Read the model definition and answer for the solid it produces. Units are mm, in the model's axes. Give positions to 0.01 mm unless a question says otherwise; leave off trailing zeros. Order: outer loops, then holes, each group sorted by start corner. A loop starts at its lowest first (then second) coordinate and runs counter-clockwise, first axis right, second up. Notation, with made-up numbers: (38.25, 79.5) - (43.25, 79.5) arc R12 ccw to (43.25, 84.5) - close; hole circle Ø2 at (-18.75, 21.25). An arc over 180 degrees is marked (long way). Return JSON: item names as keys, results as strings.
```python
from build123d import *

# Parameters (mm, degrees)
F0_R     = 3.5
F0_W     = 5
F0_H     = 25
F1_DEPTH = 1


with BuildPart() as f1:
    # F0 (on Top) → F1 (new body)
    with BuildSketch(Plane.XY):
        with BuildLine():
            ThreePointArc((24.235588, 30.946928), (30.976758, 28.377192), (35.314001, 34.142193))
            ThreePointArc((35.314001, 34.142193), (31.334351, 39.791811), (24.674606, 37.946928))
            ThreePointArc((24.674606, 37.946928), (23.325767, 34.517756), (24.235588, 30.946928))
        make_face()
        with Locations((29.314001, 34.142193)):
            Circle(F0_R, mode=Mode.SUBTRACT)
        with BuildLine():
            ThreePointArc((24.235588, 30.946928), (23.325767, 34.517756), (24.674606, 37.946928))
            Line((24.674606, 37.946928), (0, 37.946928))
            Line((0, 37.946928), (-24.674606, 37.946928))
            ThreePointArc((-24.674606, 37.946928), (-23.664383, 36.162543), (-23.314001, 34.142193))
            ThreePointArc((-23.314001, 34.142193), (-23.549, 32.479436), (-24.235588, 30.946928))
            Line((-24.235588, 30.946928), (-4.218093, 30.946928))
            Line((-4.218093, 30.946928), (-4.218093, 20.946928))
            Line((-4.218093, 20.946928), (-14.650477, 20.946928))
            Line((-14.650477, 20.946928), (-14.650477, 0))
            Line((-14.650477, 0), (-14.650477, -20.946928))
            Line((-14.650477, -20.946928), (-4.218093, -20.946928))
            Line((-4.218093, -20.946928), (-4.218093, -30.946928))
            Line((-4.218093, -30.946928), (-24.235588, -30.946928))
            ThreePointArc((-24.235588, -30.946928), (-23.549, -32.479436), (-23.314001, -34.142193))
            ThreePointArc((-23.314001, -34.142193), (-23.664383, -36.162543), (-24.674606, -37.946928))
            Line((-24.674606, -37.946928), (0, -37.946928))
            Line((0, -37.946928), (24.674606, -37.946928))
            ThreePointArc((24.674606, -37.946928), (23.325767, -34.517756), (24.235588, -30.946928))
            Line((24.235588, -30.946928), (4.218093, -30.946928))
            Line((4.218093, -30.946928), (4.218093, -20.946928))
            Line((4.218093, -20.946928), (14.650477, -20.946928))
            Line((14.650477, -20.946928), (14.650477, 0))
            Line((14.650477, 0), (14.650477, 20.946928))
            Line((14.650477, 20.946928), (4.218093, 20.946928))
            Line((4.218093, 20.946928), (4.218093, 30.946928))
            Line((4.218093, 30.946928), (24.235588, 30.946928))
        make_face()
        with Locations((-4, 0)):
            Rectangle(F0_W, F0_H, mode=Mode.SUBTRACT)
        with Locations((4, 0)):
            Rectangle(F0_W, F0_H, mode=Mode.SUBTRACT)
        with BuildLine():
            ThreePointArc((-23.314001, 34.142193), (-23.664383, 36.162543), (-24.674606, 37.946928))
            ThreePointArc((-24.674606, 37.946928), (-35.302236, 33.76663), (-24.235588, 30.946928))
            ThreePointArc((-24.235588, 30.946928), (-23.549, 32.479436), (-23.314001, 34.142193))
        make_face()
        with Locations((-29.314001, 34.142193)):
            Circle(F0_R, mode=Mode.SUBTRACT)
        with BuildLine():
            ThreePointArc((35.314001, -34.142193), (30.976758, -28.377192), (24.235588, -30.946928))
            ThreePointArc((24.235588, -30.946928), (23.325767, -34.517756), (24.674606, -37.946928))
            ThreePointArc((24.674606, -37.946928), (31.334351, -39.791811), (35.314001, -34.142193))
        make_face()
        with Locations((29.314001, -34.142193)):
            Circle(F0_R, mode=Mode.SUBTRACT)
        with BuildLine():
            ThreePointArc((-23.314001, -34.142193), (-23.549, -32.479436), (-24.235588, -30.946928))
            ThreePointArc((-24.235588, -30.946928), (-35.302236, -33.76663), (-24.674606, -37.946928))
            ThreePointArc((-24.674606, -37.946928), (-23.664383, -36.162543), (-23.314001, -34.142193))
        make_face()
        with Locations((-29.314001, -34.142193)):
            Circle(F0_R, mode=Mode.SUBTRACT)
    extrude(amount=F1_DEPTH)


solid = f1.part
```
Q1. A cutting plane is placed at C-C (z = 0.4). Give the number of separate pieces and of enclosed holes in the cut face, and give its area (3 significant figures).
Values:
{"separate pieces": "1", "enclosed holes": "6", "area": "2,110 mm²"}
Q2. A cutting plane is placed at A-A (x = 18.5). Write down the section's boundary in (y, z).
Values:
{"outline": "(-37.95, 0) - (-30.95, 0) - (-30.95, 1) - (-37.95, 1) - close; (30.95, 0) - (37.95, 0) - (37.95, 1) - (30.95, 1) - close"}
Q3. Consider L1, parallel to Y at x = 11.5, z = 0.75; L2, parallel to X at y = 7.5, z = 0.1; L3, parallel to X at y = 34, z = 0.4. Determine where each line is inside the solid, lowest interval first.
Values:
{"L1": "y = -37.95 to -30.95, -20.95 to 20.95, 30.95 to 37.95", "L2": "x = -14.65 to -6.5, -1.5 to 1.5, 6.5 to 14.65", "L3": "x = -35.31 to -32.81, -25.82 to 25.82, 32.81 to 35.31"}
Q4. A cutting plane is placed at D-D (x = 29.5). Write down the section's boundary in (y, z), and give its area (3 significant figures).
Values:
{"outline": "(-40.14, 0) - (-37.64, 0) - (-37.64, 1) - (-40.14, 1) - close; (-30.65, 0) - (-28.15, 0) - (-28.15, 1) - (-30.65, 1) - close; (28.15, 0) - (30.65, 0) - (30.65, 1) - (28.15, 1) - close; (37.64, 0) - (40.14, 0) - (40.14, 1) - (37.64, 1) - close", "area": "10.0 mm²"}
Q5. Determine the mould class of faces 1 (the flat face through (0, 1, 1)), 2 (the cylindrical face through (-25.976, -33.091, 0.493)) for opening direction X: released by +X, released by -X, zero draft, split by the parting line, or undercut.
Values:
{"face 1": "zero draft", "face 2": "undercut"}
Q6. A cutting plane is placed at B-B (y = 7). Write down the section's boundary in (x, z).
Values:
{"outline": "(-14.65, 0) - (-6.5, 0) - (-6.5, 1) - (-14.65, 1) - close; (-1.5, 0) - (1.5, 0) - (1.5, 1) - (-1.5, 1) - close; (6.5, 0) - (14.65, 0) - (14.65, 1) - (6.5, 1) - close"}
Q7. Given pin 1 (0.5 mm diameter, centred on x = 4.5, z = 0.5, fed in from +Y); pin 2 (6.5 mm diameter, centred on x = -29.31, y = 34.14, fed in from +Z); pin 3 (0.5 mm diameter, centred on y = -1.5, z = 0.5, fed in from -X), each flat-ended and moving along its own axis, determine where each tip first touches the part or whether it passes through.
Values:
{"pin 1": "stops at y = 37.95", "pin 2": "passes through", "pin 3": "stops at x = -14.65"}
